Answer from the drawing. Dimensions are ordinates in mm from the lowest x, y and z of the part. Give positions to 0.01 mm unless a question says otherwise; leave off trailing zeros. Write each loop counter-clockwise with the first axis right and the second up, starting at its lowest first coordinate (ties: lowest second). Pieces come first, ordered by that corner, then holes. Notation, with made-up numbers: (31.25, 24) -> (36.25, 24) arc R11 ccw to (36.25, 34) -> close; hole circle Ø5 at (78, 27). An arc over 180 degrees is marked (long way). Write item = value, one per line.
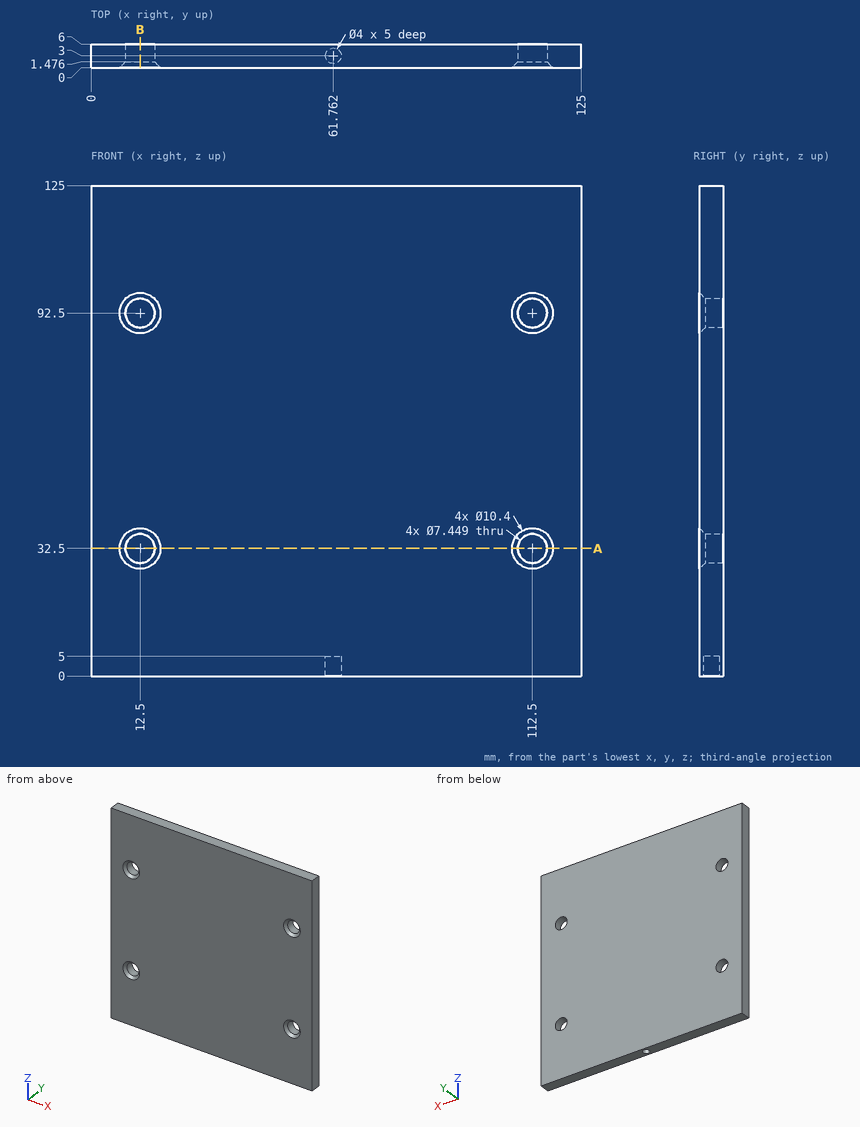
(1) Consider L1, parallel to X at y = 3, z = 32.5 (1 decimal); L2, parallel to Z at x = 111.5, y = 4.75; L3, parallel to Z at x = 14, y = 1.6. Determine where each line is inside the solid, lowest interval first.
Checks:
L1 = 0 to 8.8, 16.2 to 108.8, 116.2 to 125
L2 = 0 to 28.91, 36.09 to 88.91, 96.09 to 125
L3 = 0 to 29.09, 35.91 to 89.09, 95.91 to 125
(2) The part is cut by section B-B on x = 12.5. Determine the outline of the cut face in (y, z) (1 decimal).
Checks:
outline = (0, 0) -> (6, 0) -> (6, 28.8) -> (1.5, 28.8) -> (0, 27.3) -> close; (0, 37.7) -> (1.5, 36.2) -> (6, 36.2) -> (6, 88.8) -> (1.5, 88.8) -> (0, 87.3) -> close; (0, 97.7) -> (1.5, 96.2) -> (6, 96.2) -> (6, 125) -> (0, 125) -> close
(3) The part is cut by section A-A on z = 32.5. Determine the outline of the cut face in (x, y) (1 decimal).
Checks:
outline = (0, 0) -> (7.3, 0) -> (8.8, 1.5) -> (8.8, 6) -> (0, 6) -> close; (16.2, 1.5) -> (17.7, 0) -> (107.3, 0) -> (108.8, 1.5) -> (108.8, 6) -> (16.2, 6) -> close; (116.2, 1.5) -> (117.7, 0) -> (125, 0) -> (125, 6) -> (116.2, 6) -> close
